Verification items for the finished model (mm, model axes). A direction names the side the tool comes from. Give positions to 0.01 mm unless a question says otherwise; leave off trailing zeros. Write each loop counter-clockwise with the first axis right and the second up, starting at its lowest first coordinate (ties: lowest second). Pieces come first, ordered by that corner, then holes. Notation, with made-up numbers: M 12.5,-13.5 L 18.5,-13.5 A18 ccw 18.5,1.5 Z; hole C -37,26 d6. An arc over 180 degrees is marked long. Write item = value, one per line.
from build123d import *

# Parameters (mm, degrees)
CUT_EXTRUDE1_DEPTH      = 860.594090254
CUT_EXTRUDE1_DEPTH_BACK = 860.594090254
SKETCH2_R               = 21


with BuildPart() as part:
    # Sketch1 → Revolve1 (revolve)
    with BuildSketch(Plane.XY, mode=Mode.PRIVATE) as revolve1_sk:
        with BuildLine():
            ThreePointArc((32, 821), (22.627416998, 843.627416998), (0, 853))
            Line((0, 853), (0, 858))
            ThreePointArc((0, 858), (26.162950904, 847.162950904), (37, 821))
            Line((37, 821), (37, 40))
            Line((37, 40), (28.5, 40))
            Line((28.5, 40), (28.5, 0))
            Line((28.5, 0), (23.5, 0))
            Line((23.5, 0), (23.5, 45))
            Line((23.5, 45), (32, 45))
            Line((32, 45), (32, 821))
        make_face()
    revolve(revolve1_sk.sketch.rotate(Axis((0, 0, 0), (0, 1, 0)), 90), axis=Axis((0, 0, 0), (0, 1, 0)))

    # Sketch2 → Cut-Extrude1 (cut, two sides: drawn at the far end of the back side and taken through both)
    with BuildSketch(Plane.XY.offset(-CUT_EXTRUDE1_DEPTH_BACK)):
        with Locations((0, 821)):
            Circle(SKETCH2_R)
    extrude(amount=CUT_EXTRUDE1_DEPTH + CUT_EXTRUDE1_DEPTH_BACK, mode=Mode.SUBTRACT)


solid = part.part
1) Cross-section at C-C on y = 404.5. Record the boundary of the cut face in (x, z).
From the geometry:
outline = C 0,0 d74; hole C 0,0 d64
2) Cross-section at B-B on z = 0. Record the boundary of the cut face in (x, y), plus the area to 3 significant figures.
From the geometry:
outline = M -37,40 L -28.5,40 L -28.5,0 L -23.5,0 L -23.5,45 L -32,45 L -32,821 A32 cw 32,821 L 32,45 L 23.5,45 L 23.5,0 L 28.5,0 L 28.5,40 L 37,40 L 37,821 A37 ccw -37,821 Z
area = 8,840 mm^2
3) Depth check by flat-ended pin: P1, Ø1, axis at x = 6.5, z = 13.5, coming from the -Y side; P2, Ø4, axis at x = 14.5, z = 8, coming from the +Y side; P3, Ø8, axis at y = 117.5, z = 5.5, coming from the +X side. Enter the tip coordinate at first touch or a pass-through.
From the geometry:
P1 = 849
P2 = 855.01
P3 = 36.97
4) Tool access check on faces 1 (the cylindrical face through (31.24, 438.43, 6.94)), 2 (the cylindrical face through (-15.48, 835.19, -29.23)), 3 (the flat face through (22, 40, -19)). Record the directions out of +Z, -Z, +X, -X, +Y, -Y that give a thin tool (end or side, any length) a straight path to the whole face; none if there is none.
From the geometry:
face_1 = none
face_2 = +Z, -Z
face_3 = -Y
5) Cross-section at A-A on x = 0. Record the boundary of the cut face in (y, z), plus the area to 3 significant figures.
From the geometry:
outline = M 0,-28.5 L 40,-28.5 L 40,-37 L 800,-37 L 800,-32 L 45,-32 L 45,-23.5 L 0,-23.5 Z; M 0,23.5 L 45,23.5 L 45,32 L 800,32 L 800,37 L 40,37 L 40,28.5 L 0,28.5 Z; M 842,-30.46 A37 ccw 842,30.46 L 842,24.15 A32 cw 842,-24.15 Z
area = 8,400 mm^2
6) Material ranges on probe 1 along Z at (x, y) = (2, 196.5); probe 2 along X at (y, z) = (173.5, 1.5); probe 3 along X at (y, z) = (35, 0), recorded low to high. Write a range as from..to.
From the geometry:
probe_1 = -36.95..-31.94, 31.94..36.95
probe_2 = -36.97..-31.96, 31.96..36.97
probe_3 = -28.5..-23.5, 23.5..28.5
7) Draft check along Z on faces 4 (the flat face through (-23.4, 0, -4.1)), 5 (the cylindrical face through (-23.3, 22.82, 3.06)), 6 (the cylindrical face through (32.825, 425.033, -17.073)). Enter one of: +Z half, -Z half, draft (parallel to the pull), parting line (faces both ways), or undercut.
From the geometry:
face_4 = draft
face_5 = undercut
face_6 = parting line
